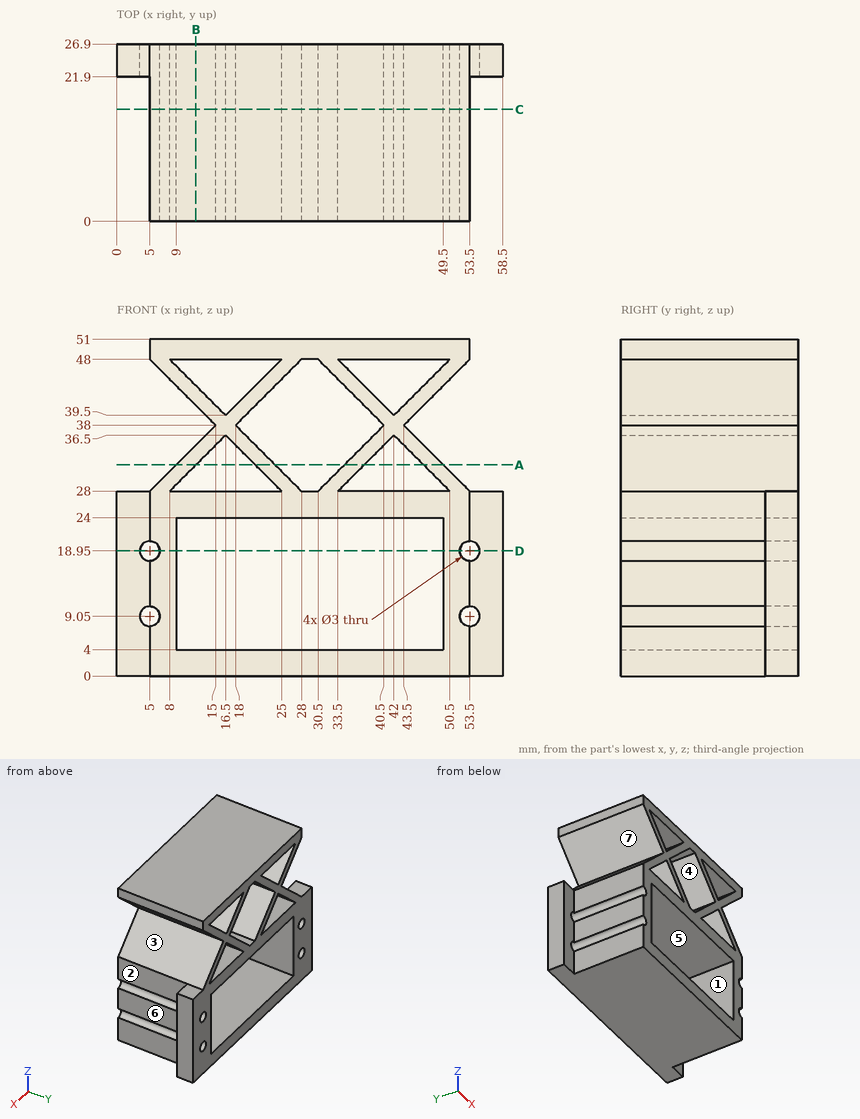
Study the drawing (mm; zero at the part's minimum x, y, z) and answer. A direction names the side the tool comes from. Coordinates: 2 decimals unless noted, no trailing zeros. Write each loop counter-clockwise with the first axis right and the second up, starting at its lowest first coordinate (ties: lowest second). Pieces come first, ordered by that corner, then holes. Notation, with made-up numbers: (28.25, 38) - (36.25, 38) arc R7 ccw to (36.25, 49) - close; hole circle Ø1 at (75, 86.25). An arc over 180 degrees is marked (long way). Return JSON: item names as keys, results as strings. Group by question number.
1. A cutting plane is placed at D-D, the plane z = 18.95. Determine the outline of the cut face in (x, y), plus the area to 4 significant figures.
2. A cutting plane is placed at B-B, the plane x = 12. Determine the outline of the cut face in (y, z).
3. Determine the mould class of the marked faces 4, 5, 6 and 7 for opening direction X: released by +X, released by -X, zero draft, split by the parting line, or undercut.
4. Which of the six approach directions +Z, -Z, +X, -X, +Y, -Y give full straight-line access (tool end or side, diameter ignored) to the marked faces 1, 2 and 3?
5. A cutting plane is placed at C-C, the plane y = 17. Give the number of separate pieces and of enclosed holes in the cut face, plus the area to 3 significant figures.
6. Straight lines are drawn through the part: L1, parallel to Z at x = 29, y = 13; L2, parallel to X at y = 8.5, z = 11; L3, parallel to X at y = 7, z = 9.05. For each, find the intervals that lie inside material, in ascending order.
7. A cutting plane is placed at A-A, the plane z = 32. Determine the outline of the cut face in (x, y).
8. Given pin 1 (2.5 mm diameter, centred on x = 53.5, z = 9.05, fed in from +Y); pin 2 (7.5 mm diameter, centred on y = 13, z = 15.5, fed in from -X); pin 3 (8 mm diameter, centred on y = 19, z = 40, fed in from -X); pin 4 (2.5 mm diameter, centred on y = 8.5, z = 22.5, fed in from +X), each flat-ended and moving along its own axis, determine where each tip first touches the part or whether it passes through.
Ans:
{
 "1": {"outline": "(0, 21.9) - (3.5, 21.9) - (3.5, 26.9) - (0, 26.9) - close; (6.5, 0) - (9, 0) - (9, 26.9) - (6.5, 26.9) - close; (49.5, 0) - (52, 0) - (52, 26.9) - (49.5, 26.9) - close; (55, 21.9) - (58.5, 21.9) - (58.5, 26.9) - (55, 26.9) - close", "area": "169.5 mm²"},
 "2": {"outline": "(0, 0) - (26.9, 0) - (26.9, 4) - (0, 4) - close; (0, 24) - (26.9, 24) - (26.9, 28) - (0, 28) - close; (0, 32) - (26.9, 32) - (26.9, 35) - (0, 35) - close; (0, 41) - (26.9, 41) - (26.9, 44) - (0, 44) - close; (0, 48) - (26.9, 48) - (26.9, 51) - (0, 51) - close"},
 "3": {"face 4": "undercut", "face 5": "undercut", "face 6": "released by +X", "face 7": "released by -X"},
 "4": {"face 1": "+Y, -Y", "face 2": "+Z, -Z, +X, -Y", "face 3": "+X, +Y, -Y"},
 "5": {"separate pieces": "1", "enclosed holes": "6", "area": "910 mm²"},
 "6": {"L1": "0 to 4, 24 to 28, 48 to 51", "L2": "5 to 9, 49.5 to 53.5", "L3": "6.5 to 9, 49.5 to 52"},
 "7": {"outline": "(9, 0) - (12, 0) - (12, 26.9) - (9, 26.9) - close; (21, 0) - (24, 0) - (24, 26.9) - (21, 26.9) - close; (34.5, 0) - (37.5, 0) - (37.5, 26.9) - (34.5, 26.9) - close; (46.5, 0) - (49.5, 0) - (49.5, 26.9) - (46.5, 26.9) - close"},
 "8": {"pin 1": "through", "pin 2": "x = 5", "pin 3": "x = 9", "pin 4": "x = 53.5"}
}
